from build123d import *

# Parameters (mm, degrees)
CROQUIS1_W              = 51
CROQUIS1_H              = 17
SALIENTE_EXTRUIR1_DEPTH = 17
CROQUIS2_W              = 15
CROQUIS2_H              = 16
CORTAR_EXTRUIR1_DEPTH   = 17
CROQUIS3_W              = 43
CROQUIS3_H              = 10
CORTAR_EXTRUIR2_DEPTH   = 16
CROQUIS6_W              = 50.5
CROQUIS6_H              = 1.5
CORTAR_EXTRUIR4_DEPTH   = 16
CORTAR_EXTRUIR5_START   = -17
CROQUIS7_W              = 6
CROQUIS7_H              = 6
CROQUIS7_W_2            = 20
CROQUIS7_H_2            = 7
CORTAR_EXTRUIR5_DEPTH   = 17
CORTAR_EXTRUIR6_START   = -39
CROQUIS8_W              = 10
CROQUIS8_H              = 6
CORTAR_EXTRUIR6_DEPTH   = 39
CROQUIS10_W             = 17
CROQUIS10_H             = 11
SALIENTE_EXTRUIR4_DEPTH = 1
CROQUIS11_W             = 17
CROQUIS11_H             = 11
SALIENTE_EXTRUIR5_DEPTH = 1
CORTAR_EXTRUIR7_START   = -17
CORTAR_EXTRUIR7_DEPTH   = 17
CROQUIS13_W             = 9.5
CROQUIS13_H             = 6
CORTAR_EXTRUIR8_DEPTH   = 7
SALIENTE_EXTRUIR6_DEPTH = 3
CROQUIS16_W             = 20
CROQUIS16_H             = 4
SALIENTE_EXTRUIR7_DEPTH = 6
CROQUIS17_R             = 1.5
CORTAR_EXTRUIR9_DEPTH   = 4
CROQUIS20_W             = 20
CROQUIS20_H             = 9.628571429
SALIENTE_EXTRUIR8_DEPTH = 0.75
CROQUIS21_W             = 20
CROQUIS21_H             = 9.628571429
SALIENTE_EXTRUIR9_DEPTH = 0.75
CORTAR_EXTRUIR10_START  = -20
CORTAR_EXTRUIR10_DEPTH  = 20


with BuildPart() as part:
    # Croquis1 → Saliente-Extruir1 (new body)
    with BuildSketch(Plane.XY):
        with Locations((-29.407991935, 18.612308998)):
            Rectangle(CROQUIS1_W, CROQUIS1_H)
    extrude(amount=SALIENTE_EXTRUIR1_DEPTH)

    # Croquis2 → Cortar-Extruir1 (cut)
    with BuildSketch(Plane.XZ.offset(-10.112308998)):
        with Locations((-29.407991935, 9)):
            Rectangle(CROQUIS2_W, CROQUIS2_H)
    extrude(amount=-CORTAR_EXTRUIR1_DEPTH, mode=Mode.SUBTRACT)

    # Croquis3 → Cortar-Extruir2 (cut)
    with BuildSketch(Plane.XY.offset(17)):
        with Locations((-29.407991935, 15.112308998)):
            Rectangle(CROQUIS3_W, CROQUIS3_H)
    extrude(amount=-CORTAR_EXTRUIR2_DEPTH, mode=Mode.SUBTRACT)

    # Croquis6 → Cortar-Extruir4 (cut)
    with BuildSketch(Plane.XY.offset(17)):
        with Locations((-29.407991935, 18.362308998)):
            Rectangle(CROQUIS6_W, CROQUIS6_H)
    extrude(amount=-CORTAR_EXTRUIR4_DEPTH, mode=Mode.SUBTRACT)

    # Croquis7 → Cortar-Extruir5 (cut)
    with BuildSketch(Plane.XY.offset(17).offset(CORTAR_EXTRUIR5_START)):
        with Locations((-6.907991935, 24.112308998)):
            Rectangle(CROQUIS7_W, CROQUIS7_H)
        with Locations((-51.907991935, 24.112308998)):
            Rectangle(CROQUIS7_W, CROQUIS7_H)
        with Locations((-29.407991935, 23.612308998)):
            Rectangle(CROQUIS7_W_2, CROQUIS7_H_2)
    extrude(amount=CORTAR_EXTRUIR5_DEPTH, mode=Mode.SUBTRACT)

    # Croquis8 → Cortar-Extruir6 (cut)
    with BuildSketch(Plane(origin=(-9.907991935, 0, 0), x_dir=(0, 0, -1), z_dir=(1, 0, 0)).offset(CORTAR_EXTRUIR6_START)):
        with Locations((-5, 24.112308998)):
            Rectangle(CROQUIS8_W, CROQUIS8_H)
    extrude(amount=CORTAR_EXTRUIR6_DEPTH, mode=Mode.SUBTRACT)

    # Croquis10 → Saliente-Extruir4 (add)
    with BuildSketch(Plane.ZY.offset(54.907991935)):
        with Locations((8.5, 15.612308998)):
            Rectangle(CROQUIS10_W, CROQUIS10_H)
    extrude(amount=SALIENTE_EXTRUIR4_DEPTH)

    # Croquis11 → Saliente-Extruir5 (add)
    with BuildSketch(Plane(origin=(-3.907991935, 0, 0), x_dir=(0, 0, -1), z_dir=(1, 0, 0))):
        with Locations((-8.5, 15.612308998)):
            Rectangle(CROQUIS11_W, CROQUIS11_H)
    extrude(amount=SALIENTE_EXTRUIR5_DEPTH)

    # Croquis12 → Cortar-Extruir7 (cut)
    with BuildSketch(Plane.XY.offset(17).offset(CORTAR_EXTRUIR7_START)):
        Polygon((-55.907991935, 21.112308998), (-51.907991935, 21.112308998), (-55.907991935, 19.740880427), align=None)
        Polygon((-2.907991935, 21.112308998), (-6.907991935, 21.112308998), (-2.907991935, 19.740880427), align=None)
    extrude(amount=CORTAR_EXTRUIR7_DEPTH, mode=Mode.SUBTRACT)

    # Croquis13 → Cortar-Extruir8 (cut)
    with BuildSketch(Plane.XY.offset(17)):
        with Locations((-44.157991935, 24.112308998)):
            Rectangle(CROQUIS13_W, CROQUIS13_H)
        with Locations((-14.657991935, 24.112308998)):
            Rectangle(CROQUIS13_W, CROQUIS13_H)
    extrude(amount=-CORTAR_EXTRUIR8_DEPTH, mode=Mode.SUBTRACT)

    # Croquis14 → Saliente-Extruir6 (add)
    with BuildSketch(Plane(origin=(0, 0, 0), x_dir=(-1, 0, 0), z_dir=(0, 0, -1))):
        Polygon((55.907991935, 10.112308998), (55.907991935, 19.740880427), (51.907991935, 21.112308998), (39.407991935, 21.112308998), (39.407991935, 20.112308998), (19.407991935, 20.112308998), (19.407991935, 21.112308998), (6.907991935, 21.112308998), (2.907991935, 19.740880427), (2.907991935, 10.112308998), align=None)
    extrude(amount=SALIENTE_EXTRUIR6_DEPTH)

    # Croquis16 → Saliente-Extruir7 (add)
    with BuildSketch(Plane(origin=(0, 20.112308998, 0), x_dir=(1, 0, 0), z_dir=(0, 1, 0))):
        with Locations((-29.407991935, 1)):
            Rectangle(CROQUIS16_W, CROQUIS16_H)
    extrude(amount=SALIENTE_EXTRUIR7_DEPTH)

    # Croquis17 → Cortar-Extruir9 (cut)
    with BuildSketch(Plane.XY.offset(1)):
        with Locations((-22.407991935, 23.612308998)):
            Circle(CROQUIS17_R)
        with Locations((-36.407991935, 23.612308998)):
            Circle(CROQUIS17_R)
    extrude(amount=-CORTAR_EXTRUIR9_DEPTH, mode=Mode.SUBTRACT)

    # Croquis20 → Saliente-Extruir8 (add)
    with BuildSketch(Plane.ZY.offset(55.907991935)):
        with Locations((7, 14.926594713)):
            Rectangle(CROQUIS20_W, CROQUIS20_H)
    extrude(amount=SALIENTE_EXTRUIR8_DEPTH)

    # Croquis21 → Saliente-Extruir9 (add)
    with BuildSketch(Plane(origin=(-2.907991935, 0, 0), x_dir=(0, 0, -1), z_dir=(1, 0, 0))):
        with Locations((-7, 14.926594713)):
            Rectangle(CROQUIS21_W, CROQUIS21_H)
    extrude(amount=SALIENTE_EXTRUIR9_DEPTH)

    # Croquis22 → Cortar-Extruir10 (cut)
    with BuildSketch(Plane.XY.offset(17).offset(CORTAR_EXTRUIR10_START)):
        Polygon((-56.657991935, 19.48373757), (-56.657991935, 19.740880427), (-55.907991935, 19.740880427), align=None)
        Polygon((-2.157991935, 19.48373757), (-2.157991935, 19.740880427), (-2.907991935, 19.740880427), align=None)
    extrude(amount=CORTAR_EXTRUIR10_DEPTH, mode=Mode.SUBTRACT)


solid = part.part
The listing builds one solid part. Answer for the finished solid, in the listing's coordinates (mm). A direction names the side the tool comes from. Round coordinates to 2 decimals unless told otherwise and drop trailing zeros. Write each loop counter-clockwise with the first axis right and the second up, starting at its lowest first coordinate (ties: lowest second). Pieces come first, ordered by that corner, then holes. Notation, with made-up numbers: (10, 3) - (40, 3) arc R18 ccw to (40, 17) - close; hole circle Ø4 at (76.25, -38). An arc over 180 degrees is marked (long way). Use a Markdown table: item, result. Add a question column.
1. For a pull along Y with two mould halves and no side action, classify faces 5 (the face through (-39.408, 24, -1)), 6 (the face through (-6, 19.112, 9)), 7 (the face through (-13, 21.112, 7)) as +Y half, -Y half, draft (parallel to the pull), parting line (faces both ways), or undercut.
2. Flat-ended cylindrical pins translate along their axes: P1, Ø4.5, axis at y = 23.5, z = -0.5, coming from the -X side; P2, Ø3, axis at x = -15, z = 10.5, coming from the -Y side; P3, Ø1.9, axis at x = -6, z = 12.5, coming from the +Y side; P4, Ø2, axis at y = 22.5, z = 9, coming from the -X side. Find the tip coordinate at first contact, or state that the pin passes through.
3. A tool of negligible diameter and unlimited length cuts with its end or side. For faces 1 (the face through (-19.408, 24, -1)), 2 (the face through (-6, 17.612, 9)), 3 (the face through (-39.408, 20.6, 9.1)), 4 (the face through (-7.908, 14, 9)), from which of +Z, -Z, +X, -X, +Y, -Y can it reach the whole face along a straight path? Write none if from no direction.
4. Consider line 1 (X direction, y = 12.5, z = 9); line 2 (X direction, y = 18, z = 6.5); line 3 (Y direction, x = -8.5, z = 13.75). Determine where each line is inside the solid, lowest interval first.
5. The part is cut by section C-C (x = -23). Write down the section's boundary in (y, z).
6. The part is cut by section A-A (z = 15.5). Write down the section's boundary in (x, y).
7. The part is cut by section D-D (z = -1). Write down the section's boundary in (x, y), and give its area (3 significant figures).
8. The part is cut by section B-B (y = 11.5). Write down the section's boundary in (x, z).
Reported:
| question | item | result |
|---|---|---|
| 1 | face 5 | draft |
| 1 | face 6 | undercut |
| 1 | face 7 | +Y half |
| 2 | P1 | x = -39.41 |
| 2 | P2 | y = 20.11 |
| 2 | P3 | y = 21.11 |
| 2 | P4 | through |
| 3 | face 1 | +Z, -Z, +X, +Y |
| 3 | face 2 | +Z |
| 3 | face 3 | +Z, +Y, -Y |
| 3 | face 4 | +Z, -Y |
| 4 | line 1 | -56.66 to -50.91, -7.91 to -2.16 |
| 4 | line 2 | -56.66 to -54.66, -4.16 to -2.16 |
| 4 | line 3 | 20.11 to 21.11 |
| 5 | outline | (10.11, -3) - (22.23, -3) - (22.23, 1) - (10.11, 1) - close; (24.99, -3) - (26.11, -3) - (26.11, 1) - (24.99, 1) - close |
| 6 | outline | (-56.66, 10.11) - (-50.91, 10.11) - (-50.91, 17.61) - (-54.66, 17.61) - (-54.66, 19.11) - (-50.91, 19.11) - (-50.91, 20.11) - (-39.41, 20.11) - (-39.41, 21.11) - (-51.91, 21.11) - (-56.66, 19.48) - close; (-19.41, 20.11) - (-7.91, 20.11) - (-7.91, 19.11) - (-4.16, 19.11) - (-4.16, 17.61) - (-7.91, 17.61) - (-7.91, 10.11) - (-2.16, 10.11) - (-2.16, 19.48) - (-6.91, 21.11) - (-19.41, 21.11) - close |
| 7 | outline | (-56.66, 10.11) - (-2.16, 10.11) - (-2.16, 19.48) - (-6.91, 21.11) - (-19.41, 21.11) - (-19.41, 26.11) - (-39.41, 26.11) - (-39.41, 21.11) - (-51.91, 21.11) - (-56.66, 19.48) - close; hole circle Ø3 at (-36.41, 23.61); hole circle Ø3 at (-22.41, 23.61) |
| 7 | area | 678 mm^2 |
| 8 | outline | (-56.66, -3) - (-2.16, -3) - (-2.16, 17) - (-7.91, 17) - (-7.91, 1) - (-50.91, 1) - (-50.91, 17) - (-56.66, 17) - close |
